Autodesk Inventor part; units mm, degrees
ref_plane "YZ Plane" through (0, 0, 0) normal (1, 0, 0) x (0, 1, 0)
ref_plane "XZ Plane" through (0, 0, 0) normal (0, 1, 0) x (-1, 0, 0)
ref_plane "XY Plane" through (0, 0, 0) normal (0, 0, 1) x (1, 0, 0)
sketch "Sketch1" plane through (0, 0, 0) normal (0, 0, 1) x (1, 0, 0)
  line L0 (0, 0) -> (46.2, 0)
  line L1 (46.2, 0) -> (46.2, 30)
  line L2 (46.2, 30) -> (0, 30)
  line L3 (0, 30) -> (0, 0)
  dimension "d0" = 46.2
  dimension "d1" = 30
extrude "Extrusion1" add sketch "Sketch1" along normal blind 3
sketch "Sketch2" plane through (0, 0, 3) normal (0, 0, 1) x (1, 0, 0)
  line L0 (0, 0) -> (46.2, 0)
  line L1 (0, 0) -> (0, 15)
  line L2 (0, 30) -> (0, 0)
  line L3 (0, 15) -> (23.1, 15)
  line L4 (46.2, 0) -> (46.2, 30)
  line L5 (23.1, 15) -> (38.1, 15)
  line L6 (23.1, 15) -> (8.1, 15)
  circle A0 centre (8.1, 15) radius 1.5
  circle A1 centre (38.1, 15) radius 1.5
  dimension "d4" = 15
  dimension "d5" = 23.1
  dimension "d6" = 15
  dimension "d7" = 15
  dimension "d8" = 3
  dimension "d9" = 3
extrude "Extrusion2" cut sketch "Sketch2" against normal blind 3
sketch "Sketch3" plane through (0, 0, 3) normal (0, 0, 1) x (1, 0, 0)
  circle A0 centre (38.1, 15) radius 1.5
  circle A1 centre (8.1, 15) radius 1.5
  line L0 (46.2, 0) -> (46.2, 30)
  line L1 (46.2, 30) -> (0, 30)
  line L2 (0, 30) -> (0, 0)
  line L3 (0, 0) -> (46.2, 0)
  circle A2 centre (38.1, 15) radius 3.5
  line L4 (38.1, 15) -> (41.6, 15)
  line L5 (41.6, 15) -> (42.6, 15)
  line L6 (42.6, 15) -> (45.6, 15)
  line L7 (45.6, 15) -> (45.6, 30)
  line L8 (45.6, 15) -> (45.6, 0)
  line L9 (0, 0) -> (46.2, 0)
  line L10 (45.6, 0) -> (46.2, 0)
  circle A3 centre (8.1, 15) radius 3.5
  line L11 (8.1, 15) -> (4.6, 15)
  line L12 (4.6, 15) -> (1.6, 15)
  line L13 (1.6, 15) -> (1.6, 30)
  line L14 (46.2, 30) -> (0, 30)
  line L15 (1.6, 30) -> (0, 30)
  line L16 (1.6, 15) -> (1.6, 0)
  dimension "d12" = 7
  dimension "d17" = 7
  dimension "d13" = 1
  dimension "d14" = 3
  dimension "d15" = 15
  dimension "d16" = 15
  dimension "d18" = 3
extrude "Extrusion6" cut sketch "Sketch3" against normal blind 40 contours L3 L2 L1 L13 L16
sketch "Sketch6" plane through (0, 0, 3) normal (0, 0, 1) x (1, 0, 0)
  line L0 (1.6, 30) -> (1.6, 0)
  line L1 (1.6, 0) -> (46.2, 0)
  line L2 (46.2, 0) -> (46.2, 30)
  line L3 (46.2, 30) -> (1.6, 30)
  circle A0 centre (8.1, 15) radius 1.5
  circle A1 centre (38.1, 15) radius 1.5
  line L4 (1.6, 0) -> (46.2, 0)
  line L5 (46.2, 0) -> (49.2, 0)
  line L6 (49.2, 0) -> (49.2, 30)
  line L7 (49.2, 30) -> (46.2, 30)
  point P0 (0, 0)
  dimension "d33" = 3
  dimension "d34" = 30
extrude "Extrusion7" add sketch "Sketch6" against normal blind 3 contours L7 L6 L5 L2
sketch "Sketch7" plane through (0, 0, 3) normal (0, 0, 1) x (1, 0, 0)
  line L0 (1.6, 30) -> (1.6, 0)
  line L1 (1.6, 0) -> (49.2, 0)
  line L2 (49.2, 0) -> (49.2, 30)
  line L3 (49.2, 30) -> (1.6, 30)
  circle A0 centre (8.1, 15) radius 1.5
  circle A1 centre (38.1, 15) radius 1.5
  line L4 (49.2, 30) -> (49.2, 0)
  line L5 (49.2, 0) -> (46.2, 0)
  line L6 (1.6, 0) -> (49.2, 0)
  line L7 (46.2, 0) -> (46.2, 30)
  line L8 (49.2, 30) -> (1.6, 30)
  line L9 (46.2, 30) -> (49.2, 30)
  point P0 (0, 0)
  dimension "d37" = 3
extrude "Extrusion8" add sketch "Sketch7" along normal blind 40 contours L3 L2 L1 L7
sketch "Sketch8" plane through (46.2, 0, 3) normal (-1, 0, 0) x (0, 0, 1)
  line L0 (0, 0) -> (0, 30)
  line L1 (0, 0) -> (40, 0)
  line L2 (40, 30) -> (40, 0)
  line L3 (0, 30) -> (40, 30)
  line L4 (0, 30) -> (0, 15)
  line L5 (0, 30) -> (0, 0)
  line L6 (0, 15) -> (25, 15)
  circle A0 centre (25, 15) radius 1.5
  circle A1 centre (25, 15) radius 15
  line L7 (-3, 30) -> (40, 30)
  line L8 (40, 0) -> (-3, 0)
  point P0 (25, 30)
  point P1 (25, 0)
  point P2 (40, 15)
  point P3 (25, 0)
  point P4 (25, 30)
  dimension "d40" = 15
  dimension "d41" = 25
  dimension "d42" = 3
extrude "Extrusion9" cut sketch "Sketch8" against normal blind 40 contours A1 L2 L1 | A1 L3 L2 | A0
fillet "Fillet1" radius 4 1 edges at (46.2, 15, 3)
sketch "Sketch9" plane through (46.2, 15, 28) normal (-1, 0, 0) x (0, 0, 1)
  line L0 (-21, -15) -> (-21, 15)
  line L1 (-21, -15) -> (0, -15)
  arc A0 (0, -15) -> (0, 15) centre (0, 0) ccw
  line L2 (-21, 15) -> (0, 15)
  circle A1 centre (0, 0) radius 1.5
  line L3 (0, 0) -> (0, 7.1)
  line L4 (0, 7.1) -> (3.25, 7.1)
  line L5 (0, 7.1) -> (-3.25, 7.1)
  circle A2 centre (0, 7.1) radius 0.5
  circle A3 centre (3.25, 7.1) radius 0.5
  circle A4 centre (-3.25, 7.1) radius 0.5
  line L6 (0, 0) -> (4.7365, 0)
  line L7 (0, 0) -> (5.6569, 5.6569)
  line L8 (0, 0) -> (8, 0) construction
  circle A5 centre (0, -7.1) radius 0.5
  circle A6 centre (3.25, -7.1) radius 0.5
  circle A7 centre (-3.25, -7.1) radius 0.5
  circle A8 centre (7.1, 0) radius 0.5
  circle A9 centre (7.1, 3.25) radius 0.5
  circle A10 centre (7.1, -3.25) radius 0.5
  circle A11 centre (-7.1, -3.25) radius 0.5
  circle A12 centre (-7.1, 0) radius 0.5
  circle A13 centre (-7.1, 3.25) radius 0.5
  point P0 (-28, -15)
  dimension "d47" = 7.1
  dimension "d48" = 3.25
  dimension "d49" = 3.25
  dimension "d50" = 1
  dimension "d51" = 1
  dimension "d52" = 1
  dimension "d53" = 8
  dimension "d54" = 45
extrude "Extrusion10" cut sketch "Sketch9" against normal blind 40 contours A2 L5 L3 | L3 L4 A2 | L5 A2 L4 | A3 | A4 | A5 | A6 | A7 | A8 | A9 | A10 | A11 | A12 | A13
sketch "Sketch10" plane through (1.6, 0, 3) normal (-1, 0, 0) x (0, 0, 1)
  line L0 (-3, 0) -> (-3, 30)
  line L1 (0, 0) -> (-3, 0)
  line L2 (0, 30) -> (0, 0)
  line L3 (-3, 30) -> (0, 30)
  point P0 (-3, 0)
extrude "Extrusion11" add sketch "Sketch10" along normal blind 20
sketch "Sketch11" plane through (0, 0, 3) normal (0, 0, 1) x (1, 0, 0)
  line L0 (42.2, 30) -> (42.2, 0)
  line L1 (42.2, 30) -> (-18.4, 30)
  line L2 (-18.4, 0) -> (-18.4, 30)
  line L3 (-18.4, 0) -> (42.2, 0)
  circle A0 centre (8.1, 15) radius 1.5
  circle A1 centre (38.1, 15) radius 1.5
  line L4 (-18.4, 30) -> (49.2, 30)
  line L5 (-18.4, 30) -> (-8.2, 30)
  line L6 (-8.2, 30) -> (-8.2, 0)
  line L7 (-18.4, 0) -> (49.2, 0)
  line L8 (-8.2, 0) -> (-11.2, 0)
  line L9 (-11.2, 0) -> (-11.2, 30)
  point P0 (0, 0)
  point P1 (-8.2, 0)
  dimension "d59" = 10.2
  dimension "d60" = 3
extrude "Extrusion12" add sketch "Sketch11" along normal blind 40 contours L6 L3 L9 L1
sketch "Sketch12" plane through (-11.2, 0, 3) normal (-1, 0, 0) x (0, 0, 1)
  circle A0 centre (25, 15) radius 1.5
  arc A1 (25, 0) -> (25, 30) centre (25, 15) ccw
  line L0 (0, 30) -> (40, 30)
  line L1 (25, 30) -> (40, 30)
  line L2 (40, 30) -> (40, 0)
  line L3 (40, 30) -> (40, 0)
  line L4 (40, 0) -> (25, 0)
  point P0 (-3, 0)
  point P1 (40, 15)
extrude "Extrusion13" cut sketch "Sketch12" against normal blind 4
sketch "Sketch13" plane through (0, 0, 3) normal (0, 0, 1) x (1, 0, 0)
  line L0 (-11.2, 0) -> (-11.2, 30)
  line L1 (-11.2, 30) -> (-18.4, 30)
  line L2 (-18.4, 0) -> (-18.4, 30)
  line L3 (-18.4, 0) -> (-11.2, 0)
  point P0 (0, 0)
extrude "Extrusion14" cut sketch "Sketch13" against normal blind 4
fillet "Fillet3" radius 4 1 edges at (-8.2, 15, 3)
properties part number "acople_1"
The model under review builds one solid part; all positions refer to its coordinate system, in mm. A direction names the side the tool comes from. Round coordinates to 2 decimals unless told otherwise and drop trailing zeros. Write each loop counter-clockwise with the first axis right and the second up, starting at its lowest first coordinate (ties: lowest second). Pieces come first, ordered by that corner, then holes. Notation, with made-up numbers: (34, 77) - (38, 77) arc R27 ccw to (38, 111) - close; hole circle Ø7 at (-8, 34). An arc over 180 degrees is marked (long way). Answer as CSV lines item,"result". Start each with the question number.
(1) We need section A-A on z = 14. State the section outline as (x, y) points.
(2) Draft analysis for pull direction Y (two halves, no side actions). For faces 3 (the flat face through (-8.2, 15, 25)), 4 (the cylindrical face through (48, 15, 43)), 5 (the cylindrical face through (-9.72, 15.07, 26.5)), 6 (the flat face through (19.1, 0, 2.7)), state which applies: pulls with the +Y half, pulls with the -Y half, needs draft (parallel to the pull), parting line crosses it, or undercut.
(3) We need section B-B on x = 38.1. State the section outline as (y, z) points, plus the area to 3 significant figures.
(4) For faces 1 (the flat face through (19, 15, 3)), 2 (the flat face through (19.1, 30, 2.5)), list the 3-axis set-ups (+Z, -Z, +X, -X, +Y, -Y) from which the entire face can be reached by the end or side of a thin tool; tool diameter is ignored.
(5) For pin 1 Ø15 at (x, y) = (13, 12) entering from +Z; pin 2 Ø2.5 at (y, z) = (15, 28) entering from -X, all flat-tipped, find the tip position at first contact; note any pin that passes through.
(6) We need section C-C on y = 10.5. State the section outline as (x, z) points.
(7) To check wall thickness, follow line 1 (Y direction, x = 46.9, z = 28); line 2 (X direction, y = 17, z = 40); line 3 (Y direction, x = 47.55, z = 20.9). State the ranges of each line that lie inside material, in increasing order.
Worked answers:
1,outline,"(-11.2, 0) - (-8.2, 0) - (-8.2, 30) - (-11.2, 30) - close; (46.2, 0) - (49.2, 0) - (49.2, 30) - (46.2, 30) - close"
2,face 3,"needs draft"
2,face 4,"parting line crosses it"
2,face 5,"undercut"
2,face 6,"pulls with the -Y half"
3,outline,"(0, 0) - (13.5, 0) - (13.5, 3) - (0, 3) - close; (16.5, 0) - (30, 0) - (30, 3) - (16.5, 3) - close"
3,area,"81.0 mm²"
4,face 1,"+Z, +Y, -Y"
4,face 2,"+Z, -Z, +X, -X, +Y"
5,pin 1,"z = 3"
5,pin 2,"through"
6,outline,"(-11.2, 0) - (49.2, 0) - (49.2, 42.31) - (46.2, 42.31) - (46.2, 7) arc R4 cw to (42.2, 3) - (-4.2, 3) arc R4 cw to (-8.2, 7) - (-8.2, 42.31) - (-11.2, 42.31) - close"
7,line 1,"0 to 7.4, 8.4 to 13.5, 16.5 to 21.6, 22.6 to 30"
7,line 2,"-11.2 to -8.2, 46.2 to 49.2"
7,line 3,"0 to 11.25, 12.25 to 14.5, 15.5 to 17.75, 18.75 to 30"
